Part model, mm, in its own coordinate system. Give positions to 0.01 mm unless a question says otherwise; leave off trailing zeros. Order: outer loops, then holes, each group sorted by start corner. A loop starts at its lowest first (then second) coordinate and runs counter-clockwise, first axis right, second up. Notation, with made-up numbers: (85.25, -26.5) - (120.25, -26.5) arc R25 ccw to (120.25, 5.5) - close; hole circle Ø7 at (78, -38.5). An arc over 180 degrees is marked (long way). Use one line per item in the form item = value. Start each with the question number.
1. Drill centre lines: line 1 (X direction, y = 758, z = 0); line 2 (Y direction, x = -14, z = 1); line 3 (X direction, y = 1637, z = 3). Where is each one in solid material? Low to high.
2. Band-saw the part on B-B, the plane y = 1519.5. List the corners of the cut face in (x, z).
3. Pin check, flat tips, straight feed: P1, Ø2.5, axis at y = 1715.5, z = -0.5, coming from the +X side; P2, Ø4, axis at y = 972.5, z = -1.5, coming from the +X side; P3, Ø1.5, axis at y = 12, z = -1, coming from the -X side. Stop position of each tip, or through.
from build123d import *

# Parameters (mm, degrees)
EXTRUDE_1_DEPTH          = 4
CHAMFER_1_SIZE           = 20
CHAMFER_1_SIZE2          = 34.641016151
FILLET_1_R               = 5
SKETCH_2_W               = 20
SKETCH_2_H               = 1568
CUT_EXTRUDE_1_DEPTH      = 1738.371002406
FILLET_2_R               = 20
FILLET_3_R               = 10
CUT_EXTRUDE_2_DEPTH      = 1738.371002406
CUT_EXTRUDE_2_DEPTH_BACK = 1738.371002406
FILLET_4_R               = 10
CHAMFER_START            = -30
CHAMFER_4_OUTLINE_W      = 63
CHAMFER_4_OUTLINE_H      = 8
CHAMFER_4_DEPTH          = 12.643216867
FILLET_6_R               = 30
CUT_EXTRUDE_3_DEPTH      = 1738.357188375


with BuildPart() as part:
    # Эскиз1 → Бобышка-Вытянуть1 (new, symmetric)
    with BuildSketch(Plane.XY):
        Polygon((0, 1653), (6, 1653), (6, 1643), (16, 1643), (16, 1668), (0, 1668), (0, 1737), (-35, 1737), (-35, 0), (14, 0), (14, 17), (6, 17), (6, 10), (0, 10), align=None)
    extrude(amount=EXTRUDE_1_DEPTH, both=True)

    # Фаска1
    chamfer_1_edges = [part.edges().sort_by_distance(p)[0] for p in [
        (-35, 1737, 0),
    ]]
    chamfer_1_side = [part.faces().sort_by_distance(p)[0] for p in [
        (-17.5, 1737, 0),
    ]]
    chamfer(chamfer_1_edges, length=CHAMFER_1_SIZE, length2=CHAMFER_1_SIZE2, reference=chamfer_1_side[0])

    # Скругление1
    fillet_1_edges = [part.edges().sort_by_distance(p)[0] for p in [
        (0, 1668, 0),
        (16, 1668, 0),
        (16, 1643, 0),
        (14, 17, 0),
        (14, 0, 0),
        (-35, 1702.358983849, 0),
        (-15, 1737, 0),
    ]]
    fillet(fillet_1_edges, radius=FILLET_1_R)

    # Эскиз2 → Вырез-Вытянуть1 (cut, through all)
    with BuildSketch(Plane.XY.offset(4)):
        with Locations((0, 844)):
            Rectangle(SKETCH_2_W, SKETCH_2_H)
    extrude(amount=-CUT_EXTRUDE_1_DEPTH, mode=Mode.SUBTRACT)

    # Скругление2
    # the kernel refuses this fillet: 20 mm, written as the material it takes off along each edge
    with BuildSketch(Plane(origin=(0, 1628, 47.301270189), x_dir=(0, 1, 0), z_dir=(0, 0, -1))) as fillet_2_piece_1:
        with BuildLine():
            CenterArc((17.320508076, -20), FILLET_2_R, 90, 60)
            Line((0, -10), (-0.346410162, -9.8))
            ThreePointArc((-0.346410162, -9.8), (-0.4, -5), (-0.4, 0))
            Line((-0.4, 0), (0, 0.4))
            Line((0, 0.4), (17.320508076, 0.4))
            Line((17.320508076, 0.4), (17.320508076, 0))
        make_face()
    extrude(amount=94.602540378, mode=Mode.SUBTRACT)
    with BuildSketch(Plane(origin=(0, 60, -47.301270189), x_dir=(-1, 0, 0), z_dir=(0, 0, 1))) as fillet_2_piece_2:
        with BuildLine():
            CenterArc((20, 17.320508076), FILLET_2_R, 180, 60)
            Line((0, 17.320508076), (-0.4, 17.320508076))
            Line((-0.4, 17.320508076), (-0.4, 0))
            Line((-0.4, 0), (0, -0.4))
            ThreePointArc((0, -0.4), (5, -0.4), (9.8, -0.346410162))
            Line((9.8, -0.346410162), (10, 0))
        make_face()
    extrude(amount=94.602540378, mode=Mode.SUBTRACT)

    # Скругление3
    fillet_3_edges = [part.edges().sort_by_distance(p)[0] for p in [
        (-10, 1628, 0),
        (-10, 60, 0),
    ]]
    fillet(fillet_3_edges, radius=FILLET_3_R)

    # Эскиз3 → Вырез-Вытянуть2 (cut, two sides: drawn at the far end of the back side and taken through both)
    with BuildSketch(Plane.XY.offset(4).offset(-CUT_EXTRUDE_2_DEPTH_BACK)):
        with BuildLine():
            Line((-15, 15), (-15, 0))
            Line((-15, 0), (-47.109663931, 0))
            Line((-47.109663931, 0), (-47.109663931, 63.037421146))
            Line((-47.109663931, 63.037421146), (-35, 63.037421146))
            Line((-35, 63.037421146), (-35, 25))
            Line((-35, 25), (-25, 25))
            ThreePointArc((-25, 25), (-17.928932188, 22.071067812), (-15, 15))
        make_face()
    extrude(amount=CUT_EXTRUDE_2_DEPTH + CUT_EXTRUDE_2_DEPTH_BACK, mode=Mode.SUBTRACT)

    # Скругление4
    fillet_4_edges = [part.edges().sort_by_distance(p)[0] for p in [
        (-15, 0, 0),
    ]]
    fillet(fillet_4_edges, radius=FILLET_4_R)

    # Фаска4: read off the stored shape, not the designer's step
    # Фаска4 outline → Фаска4 (cut)
    with BuildSketch(Plane(origin=(0, 0, 0), x_dir=(-0.2028847643439639, 0.9792026207057936, 0), z_dir=(0.9792026207057936, 0.2028847643439639, 0)).offset(CHAMFER_START)):
        with Locations((58.5, 0)):
            Rectangle(CHAMFER_4_OUTLINE_W, CHAMFER_4_OUTLINE_H)
    extrude(amount=CHAMFER_4_DEPTH, mode=Mode.SUBTRACT)

    # Скругление6
    fillet_6_edges = [part.edges().sort_by_distance(p)[0] for p in [
        (-22.857142857, 24.767710237, 0),
    ]]
    fillet(fillet_6_edges, radius=FILLET_6_R)

    # Эскиз4 → Вырез-Вытянуть3 (cut, through all)
    with BuildSketch(Plane(origin=(0, 0, 0), x_dir=(0, 0, -1), z_dir=(1, 0, 0))):
        Polygon((-4, 1707), (-4, 1737), (-2, 1737), align=None)
    cut_extrude_3 = extrude(amount=-CUT_EXTRUDE_3_DEPTH, mode=Mode.SUBTRACT)

    # Зеркальное отражение1: Вырез-Вытянуть3 across plane
    add(cut_extrude_3.mirror(Plane.XY), mode=Mode.SUBTRACT)


solid = part.part
From the geometry:
q1.line_1 = -35 to -10
q1.line_2 = 5.64 to 1736.63
q1.line_3 = -35 to -1.81
q2.outline = (-35, -4) - (-10, -4) - (-10, 4) - (-35, 4) - close
q3.P1 = 0
q3.P2 = -10
q3.P3 = -15
